Autodesk Inventor part; units mm, degrees
ref_plane "YZ Plane" through (0, 0, 0) normal (1, 0, 0) x (0, 1, 0)
ref_plane "XZ Plane" through (0, 0, 0) normal (0, 1, 0) x (-1, 0, 0)
ref_plane "XY Plane" through (0, 0, 0) normal (0, 0, 1) x (1, 0, 0)
ref_plane "Work Plane1" through (12.7619, -1.356, 21.3175) normal (0.3543575, 0, -0.93511) x (0, -1, 0)
sketch "Sketch1" plane through (12.7619, -1.356, 21.3175) normal (0.3543575, 0, -0.93511) x (0, -1, 0)
  line L0 (-22.86, -10.16) -> (-22.86, 10.16)
  line L1 (7.62, -10.16) -> (-22.86, -10.16)
  line L2 (-22.86, 10.16) -> (22.86, 10.16)
  line L3 (0.1143, 9.0805) -> (0.1143, 9.9695)
  line L4 (-0.7747, 9.0805) -> (0.1143, 9.0805)
  line L5 (-0.7747, 9.9695) -> (-0.7747, 9.0805)
  line L6 (0.1143, 9.9695) -> (-0.7747, 9.9695)
  line L7 (6.9723, 9.0805) -> (6.9723, 9.9695)
  line L8 (6.0833, 9.0805) -> (6.9723, 9.0805)
  line L9 (6.0833, 9.9695) -> (6.0833, 9.0805)
  line L10 (6.9723, 9.9695) -> (6.0833, 9.9695)
  line L11 (3.5433, 9.0805) -> (3.5433, 9.9695)
  line L12 (2.6543, 9.0805) -> (3.5433, 9.0805)
  line L13 (2.6543, 9.9695) -> (2.6543, 9.0805)
  line L14 (3.5433, 9.9695) -> (2.6543, 9.9695)
  line L15 (-3.3147, 9.0805) -> (-3.3147, 9.9695)
  line L16 (-4.2037, 9.0805) -> (-3.3147, 9.0805)
  line L17 (-4.2037, 9.9695) -> (-4.2037, 9.0805)
  line L18 (-3.3147, 9.9695) -> (-4.2037, 9.9695)
  circle A0 centre (21.0344, 8.4074) radius 0.7937
  circle A1 centre (21.0344, -8.4074) radius 0.7937
  circle A2 centre (-21.0344, 8.4074) radius 0.7937
  circle A3 centre (-21.0344, -8.4074) radius 0.7937
  line L19 (-4.2037, 9.9695) -> (-4.2037, 10.16)
  line L20 (-3.3147, 9.9695) -> (-3.3147, 10.16)
  line L21 (-0.7747, 9.9695) -> (-0.7747, 10.16)
  line L22 (0.1143, 9.9695) -> (0.1143, 10.16)
  line L23 (2.6543, 9.9695) -> (2.6543, 10.16)
  line L24 (3.5433, 9.9695) -> (3.5433, 10.16)
  line L25 (-22.86, -10.16) -> (7.62, -10.16)
  line L26 (7.62, -10.16) -> (7.62, 10.16)
  point P0 (-1.356, 19.4878)
  dimension "d0" = 30.48
extrude "Extrusion1" add sketch "Sketch1" along normal blind 12 contours L0 L2 L19 L17 L16 L15 L20 L21 L5 L4 L3 L22 L23 L13 L12 L11 L24 L26 L1
sketch "Sketch2" plane through (17.0142, -1.356, 10.0962) normal (0.3543575, 0, -0.93511) x (-0.93511, 0, -0.3543575)
  line L0 (9.9695, -6.0833) -> (10.1821, -6.0833)
  line L1 (10.1821, -6.0833) -> (10.1821, -6.9734)
  line L2 (10.1821, -6.9734) -> (9.9695, -6.9734)
  line L3 (9.9695, -6.9734) -> (9.9695, -6.0833)
  point P0 (19.4878, 1.356)
extrude "Extrusion2" cut sketch "Sketch2" against normal through all
sketch "Sketch3" plane through (3.2612, 2.8477, 17.7172) normal (-0.93511, 0, -0.3543575) x (-0.3543575, 0, 0.93511)
  line L0 (-12, 0) -> (-12, 18.6563)
  line L1 (-12, 15.3816) -> (-0.6665, -11.8237)
  line L2 (0, -11.8237) -> (-12, -11.8237)
  line L3 (-0.6665, -11.8237) -> (-12, -11.8237)
  line L4 (-12, -11.8237) -> (-12, 15.3816)
  point P0 (-15.4119, -2.8477)
extrude "Extrusion3" cut sketch "Sketch3" against normal through all
properties part number "USSensor Backing"
Geometry: final body of the model. Coordinates: model frame, mm. A direction names the side the tool comes from. Round coordinates to 2 decimals unless told otherwise and drop trailing zeros. Write each loop counter-clockwise with the first axis right and the second up, starting at its lowest first coordinate (ties: lowest second). Pieces come first, ordered by that corner, then holes. Notation, with made-up numbers: M 16,55.5 L 29,55.5 A13 ccw 29,60.5 Z; hole C -38.5,75.25 d11. An arc over 180 degrees is marked long. Write item = value, one per line.
Item 1: Section query A-A on x = 15. Return loops of the section in (y, z).
Findings:
outline = M -8.98,21.45 L 18.23,9.33 L 21.5,9.33 L 21.5,22.17 L -8.98,22.17 Z
Item 2: Section query B-B on y = 17.5. Return loops of the section in (x, z).
Findings:
outline = M 3.26,17.72 L 7.41,6.78 L 26.41,13.98 L 22.26,24.92 Z
Item 3: Material intervals for line 1 along X through (y, z) = (13.5, 15.75); line 2 along Z through (x, y) = (15, -4.5); line 3 along Y through (x, z) = (10.75, 13.5), sorted ascending. Write a range as [from, to].
Findings:
line_1 = [4.01, 25.74]
line_2 = [19.46, 22.17]
line_3 = [5.26, 21.5]
Item 4: Section query C-C on y = 1. Return loops of the section in (x, z).
Findings:
outline = M 3.26,17.72 L 4.97,13.21 L 23.97,20.41 L 22.26,24.92 Z
Item 5: Pull-direction query (Y, two-part tool) for faces 3 (the face through (4, -4.899, 17)), 4 (the face through (13, -8.976, 21)), 5 (the face through (3.581, -6.152, 16.873)); classes: pulls with the +Y half, pulls with the -Y half, needs draft (parallel to the pull), parting line crosses it, or undercut.
Findings:
face_3 = undercut
face_4 = pulls with the -Y half
face_5 = needs draft
Item 6: Pin query (flat end, axial travel): P1, Ø1.2, axis at x = 4, z = 15.5, coming from the -Y side; P2, Ø5, axis at x = 22.5, y = 7.5, coming from the -Z side; P3, Ø6, axis at x = 22.5, y = 5, coming from the +Z side. Return the tip coordinate at first contact, or that it passes through.
Findings:
P1 = -6.39
P2 = 15.49
P3 = 24.92
Item 7: Access query for faces 1 (the face through (22.436, 18.945, 18.657)), 2 (the face through (4.5, -0.581, 16)). Directions: +Z, -Z, +X, -X, +Y, -Y. A direction counts if a zero-diameter tool reaches every point of the face in a straight line with its end or side. Return the directions, or none.
Findings:
face_1 = none
face_2 = -Z, -X
